Work out the finished part from the listing and answer in its coordinate system (mm). A direction names the side the tool comes from. Give positions to 0.01 mm unless a question says otherwise; leave off trailing zeros. Loops run counter-clockwise (first coordinate to the right, second up) from the corner with the lowest first, then second, coordinate; pieces in that order, holes last. Notation, with made-up numbers: (-17.75, 6) - (27.25, 6) arc R28 ccw to (27.25, 38) - close; hole circle Ø10 at (-31, 38.25). An arc over 180 degrees is marked (long way). One line per item, written item: value.
from build123d import *

# Parameters (mm, degrees)
F15_R     = 2.5
F0_DEPTH  = 4
F3_W      = 2
F3_H      = 7
F4_DEPTH  = 3.5
F5_R      = 4
F6_DEPTH  = 5
F7_R      = 2
F8_DEPTH  = 13
F11_W     = 1
F11_H     = 11
F12_DEPTH = 12.5
F13_W     = 11
F13_H     = 5
F14_DEPTH = 25


with BuildPart() as f0:
    # F15 (on Front) → F0 (new body)
    with BuildSketch(Plane.XZ):
        Circle(F15_R)
    extrude(amount=F0_DEPTH)

    # F1 (on Right) → F2 (revolve)
    with BuildSketch(Plane.YZ):
        Polygon((-6, 0), (-4, 0), (-4, 2.5), (-4.702062, 3.0891), (-6, 2), align=None)
    revolve(axis=Axis((0, -8.987078, 0), (0, -1, 0)))

    # F3 (on Top) → F4 (cut, symmetric)
    with BuildSketch(Plane.XY):
        with Locations((0, -5.5)):
            Rectangle(F3_W, F3_H)
    extrude(amount=F4_DEPTH, both=True, mode=Mode.SUBTRACT)

    # F5 (on face) → F6 (join)
    with BuildSketch(Plane.XZ):
        Circle(F5_R)
    extrude(amount=-F6_DEPTH)

    # F7 (on face) → F8 (join)
    with BuildSketch(Plane(origin=(0, 5, 0), x_dir=(-1, 0, 0), z_dir=(0, 1, 0))):
        Circle(F7_R)
    extrude(amount=F8_DEPTH)

    # F9 (on Right) → F10 (revolve)
    with BuildSketch(Plane.YZ):
        Polygon((18, 2), (18, 0), (20, 0), (20, 1.5), (18.196913, 2.541013), align=None)
    revolve(axis=Axis((0, 19, 0), (0, 1, 0)))

    # F11 (on Top) → F12 (cut, symmetric)
    with BuildSketch(Plane.XY):
        with Locations((0, 16.5)):
            Rectangle(F11_W, F11_H)
    extrude(amount=F12_DEPTH, both=True, mode=Mode.SUBTRACT)

    # F13 (on Front) → F14 (cut, symmetric)
    with BuildSketch(Plane.XZ):
        with Locations((0, 4)):
            Rectangle(F13_W, F13_H)
        with Locations((0, -4)):
            Rectangle(F13_W, F13_H)
    extrude(amount=F14_DEPTH, both=True, mode=Mode.SUBTRACT)


solid = f0.part
1. Section D-D (y = 1.75) is taken. Write down the section's boundary in (x, z), and give its area (3 significant figures).
Output:
outline: (-3.71, -1.5) - (3.71, -1.5) arc R4 ccw to (3.71, 1.5) - (-3.71, 1.5) arc R4 ccw to start
area: 23.4 mm²
2. Find the intervals of material crossed by line 1 along Y through (x, z) = (2.75, 1.2); line 2 along X through (y, z) = (-2.5, -1); line 3 along X through (y, z) = (-2.75, -0.4), in increasing order.
Output:
line 1: y = -4.81 to -4.6, 0 to 5
line 2: x = -2.29 to -1, 1 to 2.29
line 3: x = -2.47 to -1, 1 to 2.47
3. Section C-C (y = 18.5) is taken. Write down the section's boundary in (x, z).
Output:
outline: (-1.83, -1.5) - (-0.5, -1.5) - (-0.5, 1.5) - (-1.83, 1.5) arc R2.37 ccw to start; (0.5, -1.5) - (1.83, -1.5) arc R2.37 ccw to (1.83, 1.5) - (0.5, 1.5) - close
4. Section A-A (y = 11.25) is taken. Write down the section's boundary in (x, z).
Output:
outline: (-1.32, -1.5) - (-0.5, -1.5) - (-0.5, 1.5) - (-1.32, 1.5) arc R2 ccw to start; (0.5, -1.5) - (1.32, -1.5) arc R2 ccw to (1.32, 1.5) - (0.5, 1.5) - close
5. Section B-B (y = 7.75) is taken. Write down the section's boundary in (x, z).
Output:
outline: (-1.32, -1.5) - (1.32, -1.5) arc R2 ccw to (1.32, 1.5) - (-1.32, 1.5) arc R2 ccw to start
6. Flat-ended cylindrical pins translate along their axes: pin 1 Ø1.6 at (x, z) = (0.5, 0.5) entering from -Y; pin 2 Ø0.6 at (x, z) = (3, 0) entering from -Y; pin 3 Ø1.5 at (y, z) = (17, 0.5) entering from -X; pin 4 Ø1.5 at (y, z) = (15.5, -0.5) entering from +X. Find the tip coordinate at first contact, or state that the pin passes through.
Output:
pin 1: stops at y = -6
pin 2: stops at y = -5.17
pin 3: stops at x = -2
pin 4: stops at x = 2
7. The mould has two halves that part along X. Classify faces 6 (the conical face through (2.733, -4.278, -0.025)), 7 (the flat face through (-0.5, 15, 0)), 8 (the cylindrical face through (-4, 2, 0)): released by +X, released by -X, zero draft, split by the parting line, or undercut.
Output:
face 6: released by +X
face 7: undercut
face 8: released by -X
8. For faces 1 (the cylindrical face through (-2.5, -2, 0)), 2 (the flat face through (-1, 20, 0)), 3 (the conical face through (-2.42, -5.5, 0.03)), 4 (the cylindrical face through (2, 11, 0)), 5 (the flat face through (0.5, 15, 0)), determine the directions among +Z, -Z, +X, -X, +Y, -Y from which every point of the face is accessible in a straight line to the end or side of a thin tool.
Output:
face 1: -X
face 2: +Z, -Z, +X, -X, +Y
face 3: -X, -Y
face 4: +X
face 5: +Z, -Z, +Y
